Source: three-view drawing plus pictorial views. Frame: mm from the lowest corner of the part. Give positions to 0.01 mm unless a question says otherwise; leave off trailing zeros. Loops run counter-clockwise (first coordinate to the right, second up) from the corner with the lowest first, then second, coordinate; pieces in that order, holes last. Notation, with made-up numbers: (9.5, 47) - (24.5, 47) arc R19 ccw to (24.5, 63) - close; hole circle Ø6 at (2, -20). An arc over 180 degrees is marked (long way). Answer in a Markdown table with one row per item.
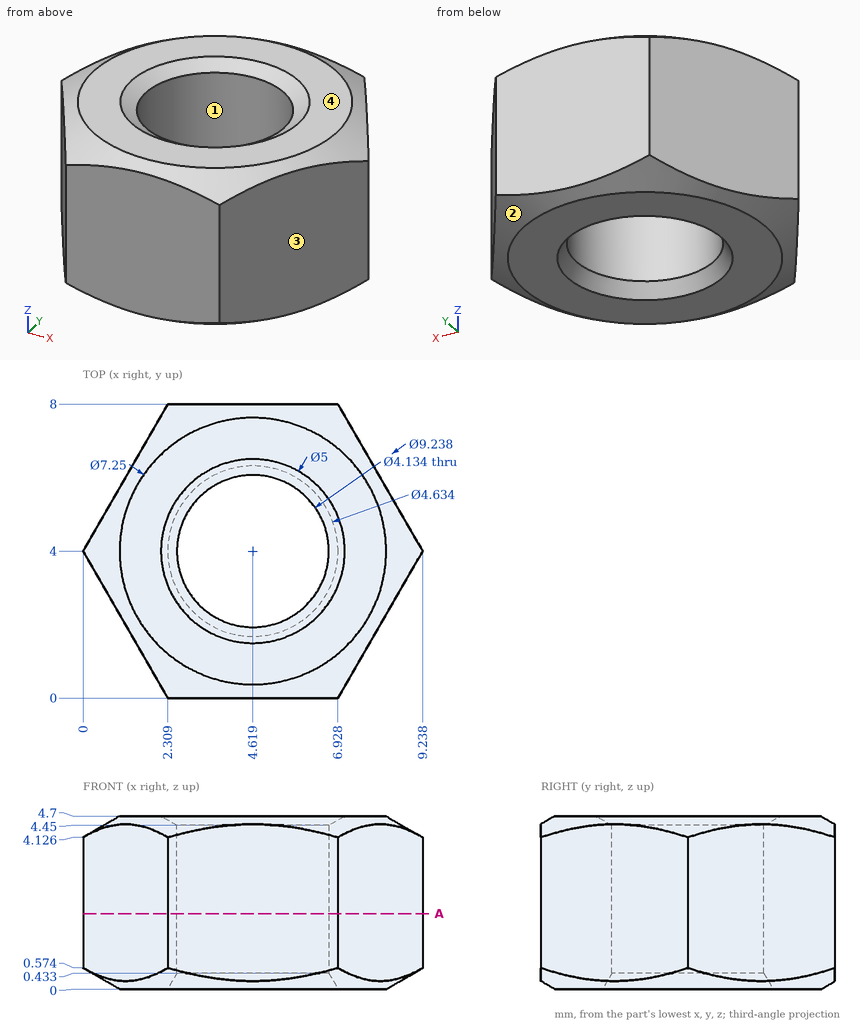
Q1. Cut plane A-A (z = 2.05). Output: boundary loops of the cut face in (x, y) (1 decimal).
Check values:
| item | result |
|---|---|
| outline | (0, 4) - (2.3, 0) - (6.9, 0) - (9.2, 4) - (6.9, 8) - (2.3, 8) - close; hole circle Ø4.1 at (4.6, 4) |
Q2. Material intervals for line 1 along Y through (x, z) = (3.25, 0.25) (1 decimal); line 2 along Y through (x, z) = (4.25, 0.6); line 3 along X through (y, z) = (2.25, 4.3) (1 decimal), sorted ascending.
Check values:
| item | result |
|---|---|
| line 1 | 0.2 to 2.3, 5.7 to 7.8 |
| line 2 | 0 to 1.97, 6.03 to 8 |
| line 3 | 1 to 3.5, 5.7 to 8.2 |
Q3. Draft query along X for the marked faces 1, 2, 3 and 4. Return one class per face: pulls with the +X half, pulls with the -X half, needs draft (parallel to the pull), parting line crosses it, or undercut.
Check values:
| item | result |
|---|---|
| face 1 | undercut |
| face 2 | parting line crosses it |
| face 3 | pulls with the +X half |
| face 4 | needs draft |
Q4. First-contact query: pin 1 (3 mm diameter, centred on x = 7.5, y = 7, fed in from +Z); pin 2 (3.5 mm diameter, centred on x = 4.62, y = 4, fed in from -Z); pin 3 (1.5 mm diameter, centred on y = 3, z = 3.5, fed in from +X). Flat tips, straight axial feed; report the tip coordinate or a pass-through.
Check values:
| item | result |
|---|---|
| pin 1 | z = 4.7 |
| pin 2 | through |
| pin 3 | x = 9.09 |
